from build123d import *

# Parameters (mm, degrees)
CROQUIS1_W              = 250
CROQUIS1_H              = 100
SALIENTE_EXTRUIR1_DEPTH = 100
VACIADO1_T              = -3
SALIENTE_EXTRUIR2_REACH = 99


with BuildPart() as part:
    # Croquis1 → Saliente-Extruir1 (new body)
    with BuildSketch(Plane.XY):
        with Locations((125, 50)):
            Rectangle(CROQUIS1_W, CROQUIS1_H)
    extrude(amount=SALIENTE_EXTRUIR1_DEPTH)

    # Vaciado1
    vaciado1_openings = [part.faces().sort_by_distance(p)[0] for p in [
        (250, 50, 50),
        (0, 50, 50),
    ]]
    offset(amount=VACIADO1_T, openings=vaciado1_openings, kind=Kind.INTERSECTION)

    # Croquis2 → Saliente-Extruir2 (add, up to next)
    with BuildSketch(Plane.XY.offset(3), mode=Mode.PRIVATE) as saliente_extruir2_sk1:
        with BuildLine():
            Line((35, 38.990872976), (111.166875619, 65.349857161))
            ThreePointArc((111.166875619, 65.349857161), (145.157572396, 67.664766629), (175.650108959, 52.46833655))
            ThreePointArc((175.650108959, 52.46833655), (178.345677223, 41.442147101), (169, 35))
            Line((169, 35), (49, 35))
            Line((49, 35), (35, 38.990872976))
        make_face()
    saliente_extruir2_tool1 = extrude(saliente_extruir2_sk1.sketch, amount=SALIENTE_EXTRUIR2_REACH, mode=Mode.PRIVATE) - part.part
    add(saliente_extruir2_tool1.solids().sort_by_distance((118.929072, 48.395279, 3))[0])


solid = part.part
Verification items for the finished model (mm, model axes). A direction names the side the tool comes from. Give positions to 0.01 mm unless a question says otherwise; leave off trailing zeros. Loops run counter-clockwise (first coordinate to the right, second up) from the corner with the lowest first, then second, coordinate; pieces in that order, holes last.
1) Thickness scan on line 1 along Y through (x, z) = (213.5, 91); line 2 along Y through (x, z) = (159, 47). Record the ranges inside material, lowest first.
2) Sectioned sample at D-D, the plane x = 52.5. Enter the section's corners in (y, z).
3) Draft check along Y on faces 1 (the flat face through (123, 51, 100)), 2 (the cylindrical face through (144.68, 67.76, 49.34)), 3 (the flat face through (123, 100, 49)). Enter one of: pulls with the +Y half, pulls with the -Y half, needs draft (parallel to the pull), parting line crosses it, or undercut.
4) Set-up check for faces 4 (the cylindrical face through (178.404, 41.601, 49.342)), 5 (the flat face through (42.098, 36.968, 49.342)), 6 (the flat face through (110, 35, 49)): record each of +Z, -Z, +X, -X, +Y, -Y from which the full face is reachable in a straight line by a thin tool's end or side.
5) Sectioned sample at A-A, the plane z = 88. Enter the section's corners in (x, y), then the cut area to 3 significant figures.
6) Sectioned sample at C-C, the plane x = 202.5. Enter the section's corners in (y, z).
7) Sectioned sample at B-B, the plane y = 93. Enter the section's corners in (x, z).
Answers:
1. line 1: y = 0 to 3, 97 to 100
1. line 2: y = 0 to 3, 35 to 63.24, 97 to 100
2. outline: (0, 0) - (100, 0) - (100, 100) - (0, 100) - close; hole (3, 3) - (35, 3) - (35, 97) - (3, 97) - close; hole (45.05, 3) - (97, 3) - (97, 97) - (45.05, 97) - close
3. face 1: needs draft
3. face 2: undercut
3. face 3: pulls with the +Y half
4. face 4: +X
4. face 5: -X
4. face 6: +X, -X
5. outline: (0, 0) - (250, 0) - (250, 3) - (0, 3) - close; (0, 97) - (250, 97) - (250, 100) - (0, 100) - close; (35, 38.99) - (49, 35) - (169, 35) arc R10 ccw to (175.65, 52.47) arc R65 ccw to (111.17, 65.35) - close
5. area: 4,750 mm2
6. outline: (0, 0) - (100, 0) - (100, 100) - (0, 100) - close; hole (3, 3) - (97, 3) - (97, 97) - (3, 97) - close
7. outline: (0, 0) - (250, 0) - (250, 3) - (0, 3) - close; (0, 97) - (250, 97) - (250, 100) - (0, 100) - close
